Check sheet for the modelled part. Datum: model origin and axes. Units: mm. A direction names the side the tool comes from. Give positions to 0.01 mm unless a question says otherwise; leave off trailing zeros. Order: outer loops, then holes, each group sorted by start corner. A loop starts at its lowest first (then second) coordinate and runs counter-clockwise, first axis right, second up. Notation, with made-up numbers: (49.25, 39.5) -> (72.25, 39.5) arc R18 ccw to (72.25, 67.5) -> close; hole circle Ø9 at (6, -19). An arc over 180 degrees is marked (long way). Answer in a Markdown table with one row per item. Add a question column.
(1) Set-up check for faces 4 (the face through (36.961, -47, -1)), 5 (the face through (2.171, -1.426, -19.249)), 6 (the face through (11.961, -30, -38)): record each of +Z, -Z, +X, -X, +Y, -Y from which the full face is reachable in a straight line by a thin tool's end or side.
(2) Thickness scan on L1, parallel to X at y = -20, z = -39; L2, parallel to X at y = -20, z = -16; L3, parallel to Z at x = 17.5, y = -14. Record the ranges inside material, lowest first. Write a range as [from, to].
(3) Cross-section at A-A (z = -35.5). Record the cut outline in (x, y).
(4) Cross-section at D-D (z = 1.5). Record the cut outline in (x, y), then the cut area to 3 significant figures.
(5) Cross-section at C-C (x = -19). Record the cut outline in (y, z).
(6) Release check for a two-part mould opening along X. For faces 1 (the face through (-46.54, -30.35, 57.82)), 2 (the face through (25, -2, 40.699)), 3 (the face through (2.171, -58.574, -19.249)) record: released by +X, released by -X, zero draft, split by the parting line, or undercut.
(7) Go/stop test with flat-tipped pins: pin 1 (1.5 mm diameter, centred on x = -11, z = -38.5, fed in from +Y); pin 2 (18 mm diameter, centred on x = -28.04, y = -20, fed in from -Z); pin 3 (9.5 mm diameter, centred on x = -20.5, z = 34, fed in from +Y). Record where each tip stops, or that it passes through.
```python
from build123d import *

# Parameters (mm, degrees)
F1_DEPTH = 60
F2_W     = 70
F2_H     = 15
F3_DEPTH = 50
F4_R     = 15
F5_R     = 15
F6_DEPTH = 67.5
F7_W     = 20
F7_H     = 12
F8_DEPTH = 5
F9_R     = 4.99999


# Not quite as in the source:
# - a fillet or chamfer is up to 0.001 mm smaller than in the source, because OpenCascade refuses the exact size


with BuildPart() as f1:
    # F0 (on Front) → F1 (new body)
    with BuildSketch(Plane.XZ):
        with BuildLine():
            Line((-8.0390890029, 59.2476050396), (-48.0390890029, 59.2476050396))
            Line((-48.0390890029, 59.2476050396), (-48.0390890029, 49.1578779955))
            ThreePointArc((-48.0390890029, 49.1578779955), (-31.8798250439, 34.2027415175), (-48.0390890029, 19.2476050396))
            Line((-48.0390890029, 19.2476050396), (-48.0390890029, -60.7523949604))
            Line((-48.0390890029, -60.7523949604), (-8.0390890029, -60.7523949604))
            Line((-8.0390890029, -60.7523949604), (-8.0390890029, -20.7523949604))
            Line((-8.0390890029, -20.7523949604), (11.9609109971, -20.7523949604))
            Line((11.9609109971, -20.7523949604), (11.9609109971, -60.7523949604))
            Line((11.9609109971, -60.7523949604), (51.9609109971, -60.7523949604))
            Line((51.9609109971, -60.7523949604), (51.9609109971, 19.2476050396))
            ThreePointArc((51.9609109971, 19.2476050396), (35.8016470382, 34.2027415175), (51.9609109971, 49.1578779955))
            Line((51.9609109971, 49.1578779955), (51.9609109971, 59.2476050396))
            Line((51.9609109971, 59.2476050396), (11.9609109971, 59.2476050396))
            Line((11.9609109971, 59.2476050396), (11.9609109971, 19.2476050396))
            Line((11.9609109971, 19.2476050396), (-8.0390890029, 19.2476050396))
            Line((-8.0390890029, 19.2476050396), (-8.0390890029, 59.2476050396))
        make_face()
    extrude(amount=F1_DEPTH)

    # F2 (on face) → F3 (cut)
    with BuildSketch(Plane.XZ.offset(60)):
        with Locations((1.9609109971, -0.7523949604)):
            Rectangle(F2_W, F2_H)
    extrude(amount=-F3_DEPTH, mode=Mode.SUBTRACT)

    # F4 (on face) + F5 (on face) → F6 (cut)
    with BuildSketch(Plane(origin=(0, 0, -60.7523949604), x_dir=(1, 0, 0), z_dir=(0, 0, -1))):
        with Locations((-28.0390890029, 20)):
            Circle(F4_R)
    with BuildSketch(Plane(origin=(0, 0, -60.7523949604), x_dir=(1, 0, 0), z_dir=(0, 0, -1))):
        with Locations((31.9609109971, 20)):
            Circle(F5_R)
    extrude(amount=-F6_DEPTH, mode=Mode.SUBTRACT)

    # F7 (on face) → F8 (cut)
    with BuildSketch(Plane.XZ):
        with BuildLine():
            Line((37.9935329711, 28.6991419792), (37.9935329711, 40.6991419792))
            Line((37.9935329711, 40.6991419792), (37.281411055, 40.6991419792))
            ThreePointArc((37.281411055, 40.6991419792), (35.811430972, 34.7444261941), (36.8477804729, 28.6991419792))
            Line((36.8477804729, 28.6991419792), (37.9935329711, 28.6991419792))
        make_face()
        with Locations((1.9609109971, 34.6991419792)):
            Rectangle(F7_W, F7_H)
        with BuildLine():
            Line((-8.0390890029, 28.6991419792), (-8.0390890029, 40.6991419792))
            Line((-8.0390890029, 40.6991419792), (-33.3595890607, 40.6991419792))
            ThreePointArc((-33.3595890607, 40.6991419792), (-31.8896089777, 34.7444261941), (-32.9259584786, 28.6991419792))
            Line((-32.9259584786, 28.6991419792), (-8.0390890029, 28.6991419792))
        make_face()
        with BuildLine():
            ThreePointArc((-32.9259584786, 28.6991419792), (-31.8896089777, 34.7444261941), (-33.3595890607, 40.6991419792))
            Line((-33.3595890607, 40.6991419792), (-38.3973060106, 40.6991419792))
            Line((-38.3973060106, 40.6991419792), (-38.3973060106, 28.6991419792))
            Line((-38.3973060106, 28.6991419792), (-32.9259584786, 28.6991419792))
        make_face()
        with BuildLine():
            ThreePointArc((36.8477804729, 28.6991419792), (35.811430972, 34.7444261941), (37.281411055, 40.6991419792))
            Line((37.281411055, 40.6991419792), (11.9609109971, 40.6991419792))
            Line((11.9609109971, 40.6991419792), (11.9609109971, 28.6991419792))
            Line((11.9609109971, 28.6991419792), (36.8477804729, 28.6991419792))
        make_face()
    extrude(amount=F8_DEPTH, mode=Mode.SUBTRACT)

    # F9 (radius 5 in the source; OpenCascade refuses exactly that, so slightly less here)
    f9_edges = [f1.edges().sort_by_distance(p)[0] for p in [
        (-31.879825, -60, 34.202742),
        (-48.039089, -60, 54.202742),
        (-28.039089, -60, 59.247605),
        (-8.039089, -60, 39.247605),
        (1.960911, -60, 19.247605),
        (11.960911, -60, 39.247605),
        (31.960911, -60, 59.247605),
        (51.960911, -60, 54.202742),
        (35.801647, -60, 34.202742),
        (51.960911, -60, -20.752395),
        (-48.039089, -60, -20.752395),
        (-28.039089, -60, -60.752395),
        (31.960911, -60, -60.752395),
        (11.960911, -60, -40.752395),
        (-8.039089, -60, -40.752395),
        (1.960911, -60, -20.752395),
        (1.960911, -60, -8.252395),
        (1.960911, -60, 6.747605),
        (51.960911, -30, 59.247605),
        (11.960911, -30, 59.247605),
        (-8.039089, -30, 59.247605),
        (-48.039089, -30, 59.247605),
        (31.960911, 0, 59.247605),
        (-28.039089, 0, 59.247605),
        (43.312591, 0, 47.199435),
        (42.848135, 0, 21.484973),
        (-38.926313, 0, 21.484973),
        (-39.390769, 0, 47.199435),
        (51.960911, 0, 54.202742),
        (-48.039089, 0, 54.202742),
        (-48.039089, 0, -20.752395),
        (51.960911, 0, -20.752395),
        (-28.039089, 0, -60.752395),
        (31.960911, 0, -60.752395),
        (-8.039089, 0, -40.752395),
        (11.960911, 0, -40.752395),
        (1.960911, 0, -20.752395),
        (11.960911, -30, -60.752395),
        (-8.039089, -30, -60.752395),
        (-48.039089, -30, -60.752395),
        (51.960911, -30, -60.752395),
    ]]
    fillet(f9_edges, radius=F9_R)


solid = f1.part
```
Answer below:
| question | item | result |
|---|---|---|
| 1 | face 4 | -Y |
| 1 | face 5 | -Z, +Y |
| 1 | face 6 | -Z, +Y, -Y |
| 2 | L1 | x = [-48.04, -43.04], [-13.04, -8.04], [11.96, 16.96], [46.96, 51.96] |
| 2 | L2 | x = [-48.04, -43.04], [-13.04, 16.96], [46.96, 51.96] |
| 2 | L3 | z = [-60.75, -8.25], [6.75, 59.25] |
| 3 | outline | (-48.04, -55) arc R5 ccw to (-43.04, -60) -> (-13.04, -60) arc R5 ccw to (-8.04, -55) -> (-8.04, -5) arc R5 ccw to (-13.04, 0) -> (-43.04, 0) arc R5 ccw to (-48.04, -5) -> close; (11.96, -55) arc R5 ccw to (16.96, -60) -> (46.96, -60) arc R5 ccw to (51.96, -55) -> (51.96, -5) arc R5 ccw to (46.96, 0) -> (16.96, 0) arc R5 ccw to (11.96, -5) -> close; hole circle Ø30 at (-28.04, -20); hole circle Ø30 at (31.96, -20) |
| 4 | outline | (-48.04, -55) arc R5 ccw to (-43.04, -60) -> (-33.04, -60) -> (-33.04, -34.14) arc R15 cw (long way) to (-16.86, -10) -> (20.78, -10) arc R15 cw (long way) to (36.96, -34.14) -> (36.96, -60) -> (46.96, -60) arc R5 ccw to (51.96, -55) -> (51.96, -5) arc R5 ccw to (46.96, 0) -> (-43.04, 0) arc R5 ccw to (-48.04, -5) -> close |
| 4 | area | 1,940 mm² |
| 5 | outline | (-60, -55.75) arc R5 ccw to (-55, -60.75) -> (-31.97, -60.75) -> (-31.97, -8.25) -> (-55, -8.25) arc R5 ccw to (-60, -13.25) -> close; (-60, 11.75) arc R5 ccw to (-55, 6.75) -> (-8.03, 6.75) -> (-8.03, -60.75) -> (-5, -60.75) arc R5 ccw to (0, -55.75) -> (0, 28.7) -> (-5, 28.7) -> (-5, 40.7) -> (0, 40.7) -> (0, 54.25) arc R5 ccw to (-5, 59.25) -> (-55, 59.25) arc R5 ccw to (-60, 54.25) -> close |
| 6 | face 1 | released by -X |
| 6 | face 2 | zero draft |
| 6 | face 3 | undercut |
| 7 | pin 1 | stops at y = -0.17 |
| 7 | pin 2 | stops at z = 6.75 |
| 7 | pin 3 | stops at y = -5 |
